```python
from build123d import *

# Parameters (mm, degrees)
SKETCH1_R           = 1.7526
SKETCH1_R_2         = 3.175
BOSS_EXTRUDE1_DEPTH = 3.175


with BuildPart() as part:
    # Sketch1 → Boss-Extrude1 (new, symmetric)
    with BuildSketch(Plane.XY):
        with BuildLine():
            Line((-16.5989, 7.309993), (12.6111, 7.309993))
            ThreePointArc((12.6111, 7.309993), (14.85616403, 6.38005703), (15.7861, 4.134993))
            Line((15.7861, 4.134993), (15.7861, -3.864460368))
            ThreePointArc((15.7861, -3.864460368), (14.85616403, -6.109524399), (12.6111, -7.039460368))
            Line((12.6111, -7.039460368), (3.2131, -7.039460368))
            ThreePointArc((3.2131, -7.039460368), (0.96803597, -7.969396338), (0.0381, -10.214460368))
            Line((0.0381, -10.214460368), (0.0381, -43.70392319))
            ThreePointArc((0.0381, -43.70392319), (0.96803597, -45.948987221), (3.2131, -46.87892319))
            Line((3.2131, -46.87892319), (18.9611, -46.87892319))
            ThreePointArc((18.9611, -46.87892319), (21.20616403, -47.80885916), (22.1361, -50.05392319))
            Line((22.1361, -50.05392319), (22.1361, -63.00792319))
            ThreePointArc((22.1361, -63.00792319), (21.20616403, -65.252987221), (18.9611, -66.18292319))
            Line((18.9611, -66.18292319), (-16.5989, -66.18292319))
            ThreePointArc((-16.5989, -66.18292319), (-18.84396403, -65.252987221), (-19.7739, -63.00792319))
            Line((-19.7739, -63.00792319), (-19.7739, 4.134993))
            ThreePointArc((-19.7739, 4.134993), (-18.84396403, 6.38005703), (-16.5989, 7.309993))
        make_face()
        with Locations((-8.6995, 0.959993)):
            Circle(SKETCH1_R, mode=Mode.SUBTRACT)
        with Locations((8.6995, 0.959993)):
            Circle(SKETCH1_R, mode=Mode.SUBTRACT)
        with Locations((-7.5819, -22.74892319)):
            Circle(SKETCH1_R, mode=Mode.SUBTRACT)
        with Locations((-7.5819, -30.36892319)):
            Circle(SKETCH1_R_2, mode=Mode.SUBTRACT)
        with Locations((-7.5819, -58.81692319)):
            Circle(SKETCH1_R, mode=Mode.SUBTRACT)
        with Locations((5.8801, -58.81692319)):
            Circle(SKETCH1_R, mode=Mode.SUBTRACT)
        with Locations((0, 0.959993)):
            Circle(SKETCH1_R, mode=Mode.SUBTRACT)
    extrude(amount=BOSS_EXTRUDE1_DEPTH, both=True)


solid = part.part
```
Check sheet for the modelled part. Datum: model origin and axes. Units: mm. A direction names the side the tool comes from. Give positions to 0.01 mm unless a question says otherwise; leave off trailing zeros. Order: outer loops, then holes, each group sorted by start corner. A loop starts at its lowest first (then second) coordinate and runs counter-clockwise, first axis right, second up. Notation, with made-up numbers: (83.25, 10.5) -> (113.25, 10.5) arc R22 ccw to (113.25, 17.5) -> close; hole circle Ø2 at (28.5, 53). An arc over 180 degrees is marked (long way). Return JSON: item names as keys, results as strings.
1. Mould release check, pull along X, two halves, no side actions. Record for faces 1 (the cylindrical face through (-7.03, 1.49, -0.04)), 2 (the cylindrical face through (-18.869, 6.355, 0.044)), 3 (the flat face through (8, -7.039, 0)): +X half, -X half, draft (parallel to the pull), parting line (faces both ways), or undercut.
From the geometry:
{"face 1": "undercut", "face 2": "-X half", "face 3": "draft"}
2. Cross-section at A-A, the plane x = -8. Record the cut outline in (y, z) (3 decimals), plus the area to 3 significant figures.
From the geometry:
{"outline": "(-66.183, -3.175) -> (-60.519, -3.175) -> (-60.519, 3.175) -> (-66.183, 3.175) -> close; (-57.115, -3.175) -> (-33.516, -3.175) -> (-33.516, 3.175) -> (-57.115, 3.175) -> close; (-27.222, -3.175) -> (-24.451, -3.175) -> (-24.451, 3.175) -> (-27.222, 3.175) -> close; (-21.047, -3.175) -> (-0.647, -3.175) -> (-0.647, 3.175) -> (-21.047, 3.175) -> close; (2.567, -3.175) -> (7.31, -3.175) -> (7.31, 3.175) -> (2.567, 3.175) -> close", "area": "363 mm^2"}
3. Go/stop test with a flat-tipped pin: P1, Ø1.9, axis at y = 1.5, z = -0.5, coming from the +X side. Record where the tip stops, or that it passes through.
From the geometry:
{"P1": "x = 15.79"}
4. Material ranges on probe 1 along X at (y, z) = (-59, 2.5); probe 2 along Y at (x, z) = (6.5, -1); probe 3 along Y at (x, z) = (-10, -2.5), recorded low to high. Write a range as [from, to].
From the geometry:
{"probe 1": "[-19.77, -9.32], [-5.84, 4.14], [7.62, 22.14]", "probe 2": "[-66.18, -60.46], [-57.18, -46.88], [-7.04, 7.31]", "probe 3": "[-66.18, -32.43], [-28.31, -0.21], [2.13, 7.31]"}
5. Cross-section at C-C, the plane y = -12. Record the cut outline in (x, z) (3 decimals).
From the geometry:
{"outline": "(-19.774, -3.175) -> (0.038, -3.175) -> (0.038, 3.175) -> (-19.774, 3.175) -> close"}
6. Cross-section at B-B, the plane z = 1.5. Count the separate pieces of the cut face and the enclosed holes in it, plus the area to 3 significant figures.
From the geometry:
{"separate pieces": "1", "enclosed holes": "7", "area": "2,010 mm^2"}
7. Cross-section at D-D, the plane x = 15. Record the cut outline in (y, z) (3 decimals), plus the area to 3 significant figures.
From the geometry:
{"outline": "(-66.183, -3.175) -> (-46.879, -3.175) -> (-46.879, 3.175) -> (-66.183, 3.175) -> close; (-5.956, -3.175) -> (6.226, -3.175) -> (6.226, 3.175) -> (-5.956, 3.175) -> close", "area": "200 mm^2"}
8. Set-up check for faces 4 (the flat face through (11, -46.879, 0)), 5 (the flat face through (1, -66.183, 0)): record each of +Z, -Z, +X, -X, +Y, -Y from which the full face is reachable in a straight line by a thin tool's end or side.
From the geometry:
{"face 4": "+Z, -Z, +X", "face 5": "+Z, -Z, +X, -X, -Y"}
